Source: CAD feature listing. Evaluate the final solid. Frame: model axes, mm. A direction names the side the tool comes from. Round coordinates to 2 decimals unless told otherwise and drop trailing zeros. Order: outer loops, then holes, each group sorted by start corner. A loop starts at its lowest first (then second) coordinate and runs counter-clockwise, first axis right, second up.
```python
from build123d import *

# Parameters (mm, degrees)
F1_DEPTH = 30
F2_R     = 1.59
F3_DEPTH = 1.331
F5_DEPTH = 0.8
F7_DEPTH = 500


with BuildPart() as f1:
    # F0 (on Top) → F1 (new body)
    with BuildSketch(Plane.XY):
        Polygon((-6.304383, 7.103708), (-6.304383, -5.596292), (-4.974383, -5.596292), (-4.974383, 5.773708), (6.590617, 5.773708), (6.590617, 7.103708), align=None)
    extrude(amount=F1_DEPTH)

    # F2 (on face) → F3 (cut, through all)
    with BuildSketch(Plane.XZ.offset(-5.773708)):
        with Locations((6.445617, 17.78)):
            Circle(F2_R)
    extrude(amount=-F3_DEPTH, mode=Mode.SUBTRACT)

    # F4 (on face) → F5 (join, symmetric)
    with BuildSketch(Plane.YZ.offset(-4.974383)):
        Polygon((1.439443, 7.189216), (-5.295732, 7.189216), (-5.407412, 0), (-4.006254, -0.653366), (-4.006254, -4.282046), (-2.106292, -4.27), (-2.106292, -0.640731), (-0.785984, 0), (1.436453, 0), align=None)
    extrude(amount=F5_DEPTH, both=True)

    # F6 (on face) → F7 (cut, symmetric)
    with BuildSketch(Plane.XZ.offset(4.006254)):
        Polygon((-4.174383, 0), (-4.974383, -1.282046), (-4.974383, -4.282046), (-4.174383, -4.282046), align=None)
    extrude(amount=F7_DEPTH, both=True, mode=Mode.SUBTRACT)

    # F8: F1 across face


with BuildPart() as f1_1:
    add(f1.part)
    add(f1.part.mirror(Plane(origin=(6.590617, 6.438708, 8.098313), x_dir=(0, 1, 0), z_dir=(1, 0, 0))))


solid = f1_1.part
```
1. Section D-D on z = 24.5. Return loops of the section in (x, y), plus the area to 3 significant figures.
2. Line query: line 1 along X through (y, z) = (3, 11); line 2 along X through (y, z) = (6.15, 17.78); line 3 along Y through (x, z) = (9.75, 11.5). Output: solid intervals per line, ascending.
3. Access query for faces 4 (the face through (18, -2, 7.189)), 5 (the face through (17.356, -2, 4)), 6 (the face through (18.5, -4.006, -2.4)), 7 (the face through (18.5, -2.106, -2.5)), 8 (the face through (17.66, -3.13, -0.49)). Directions: +Z, -Z, +X, -X, +Y, -Y. A direction counts if a zero-diameter tool reaches every point of the face in a straight line with its end or side. Return the directions, or none.
4. First-contact query: pin 1 (12 mm diameter, centred on x = 3.5, z = 1.5, fed in from -Y); pin 2 (1 mm diameter, centred on x = 18.5, z = -2, fed in from +Y); pin 3 (1 mm diameter, centred on x = -5, z = -2, fed in from -Y). Flat tips, straight axial feed; report the tip coordinate or a pass-through.
5. Section C-C on x = 5.25. Return loops of the section in (y, z).
6. Section B-B on z = 17.78. Return loops of the section in (x, y), plus the area to 3 significant figures.
7. Pull-direction query (X, two-part tool) for faces 1 (the face through (18.956, -3, -2)), 2 (the face through (4.856, 6.429, 17.817)), 3 (the face through (-5.14, -4.72, -0.32)); classes: released by +X, released by -X, zero draft, split by the parting line, or undercut.
8. Section A-A on y = 5. Return loops of the section in (x, z), plus the area to 3 significant figures.
Result:
1. outline: (-6.3, -5.6) - (-4.97, -5.6) - (-4.97, 5.77) - (18.16, 5.77) - (18.16, -5.6) - (19.49, -5.6) - (19.49, 7.1) - (-6.3, 7.1) - close
1. area: 64.5 mm2
2. line 1: x = -6.3 to -4.97, 18.16 to 19.49
2. line 2: x = -6.3 to 4.86, 8.33 to 19.49
2. line 3: y = 5.77 to 7.1
3. face 4: +Z, -Y
3. face 5: +Z, -Z, -Y
3. face 6: -Z, +X, -X, -Y
3. face 7: -Z, +X, -X, +Y
3. face 8: -Z, +Y, -Y
4. pin 1: stops at y = 5.77
4. pin 2: stops at y = -2.11
4. pin 3: stops at y = -4.01
5. outline: (5.77, 0) - (7.1, 0) - (7.1, 16.73) - (5.77, 16.73) - close; (5.77, 18.83) - (7.1, 18.83) - (7.1, 30) - (5.77, 30) - close
6. outline: (-6.3, -5.6) - (-4.97, -5.6) - (-4.97, 5.77) - (4.86, 5.77) - (4.86, 7.1) - (-6.3, 7.1) - close; (8.33, 5.77) - (18.16, 5.77) - (18.16, -5.6) - (19.49, -5.6) - (19.49, 7.1) - (8.33, 7.1) - close
6. area: 59.9 mm2
7. face 1: released by +X
7. face 2: undercut
7. face 3: zero draft
8. outline: (-6.3, 0) - (-4.97, 0) - (-4.97, 30) - (-6.3, 30) - close; (18.16, 0) - (19.49, 0) - (19.49, 30) - (18.16, 30) - close
8. area: 79.8 mm2
